from build123d import *

# Parameters (mm, degrees)
MODEL_R         = 0.5
MODEL_R_2       = 1.782992023
MODEL_R_3       = 1.590607237
MODEL_R_4       = 1.168321926
MODEL_R_5       = 1.005990221
MODEL_R_6       = 0.862372678
MODEL_R_7       = 1.386768465
MODEL_R_8       = 2.007691982
MODEL_R_9       = 2.246211192
EXTRUDE_1_DEPTH = 2


with BuildPart() as part:
    # Model → 凸台-拉伸1 (new body)
    with BuildSketch(Plane.XY):
        with BuildLine():
            Line((7.038065488, 6.287794997), (6.161323194, 8.085383089))
            Line((6.161323194, 8.085383089), (11.554087472, 10.71560997))
            Line((11.554087472, 10.71560997), (12.430829766, 8.918021877))
            Line((12.430829766, 8.918021877), (22.753800963, 13.952871341))
            Line((22.753800963, 13.952871341), (27.429909526, 30.259640434))
            ThreePointArc((27.429909526, 30.259640434), (29.651920806, 31.70137695), (31.356032886, 29.673584966))
            Line((31.356032886, 29.673584966), (31.073854544, 12.913284736))
            Line((31.073854544, 12.913284736), (84.46937713, 7.138642034))
            Line((84.46937713, 7.138642034), (76.356996628, 7.138642034))
            Line((76.356996628, 7.138642034), (76.356996628, 5.138642034))
            Line((76.356996628, 5.138642034), (84.613173024, 5.138642034))
            Line((84.613173024, 5.138642034), (84.613173024, 3.138642034))
            Line((84.613173024, 3.138642034), (39.080128632, 2.952174352))
            Line((39.080128632, 2.952174352), (6.368039675, 2.818983184))
            Line((6.368039675, 2.818983184), (6.36396809, 3.818974895))
            Line((6.36396809, 3.818974895), (1.939296742, 3.800959318))
            Line((1.939296742, 3.800959318), (7.038065488, 6.287794997))
        make_face()
        with Locations((29.356650707, 29.723293138)):
            Circle(MODEL_R, mode=Mode.SUBTRACT)
        with Locations((34.697579439, 7.654463755)):
            Circle(MODEL_R_2, mode=Mode.SUBTRACT)
        with Locations((40.228196013, 7.265180246)):
            Circle(MODEL_R_3, mode=Mode.SUBTRACT)
        with Locations((57.662403713, 6.323039134)):
            Circle(MODEL_R_4, mode=Mode.SUBTRACT)
        with Locations((61.677618383, 6.049673892)):
            Circle(MODEL_R_5, mode=Mode.SUBTRACT)
        with Locations((65.97541766, 5.870473213)):
            Circle(MODEL_R_6, mode=Mode.SUBTRACT)
        with Locations((45.214294389, 6.944127982)):
            Circle(MODEL_R_7, mode=Mode.SUBTRACT)
        with Locations((28.636152213, 7.943525557)):
            Circle(MODEL_R_8, mode=Mode.SUBTRACT)
        with Locations((22.680090468, 8.022724278)):
            Circle(MODEL_R_9, mode=Mode.SUBTRACT)
        with Locations((51.523752732, 6.556908357)):
            Circle(MODEL_R_7, mode=Mode.SUBTRACT)
    extrude(amount=EXTRUDE_1_DEPTH)


solid = part.part
Could you check a few things on this model? Use its own coordinates, in mm. A direction names the side the tool comes from. Coordinates: 2 decimals unless noted, no trailing zeros. Loops run counter-clockwise (first coordinate to the right, second up) from the corner with the lowest first, then second, coordinate; pieces in that order, holes last.
1. For faces 4 (the face through (12, 9.8, 1)), 5 (the face through (76.357, 6, 1)), 6 (the face through (6.61, 7.17, 0.99)), which set-ups out of +Z, -Z, +X, -X, +Y, -Y let a thin tool reach every point of the face, with its end or its side?
2. For P1, Ø4.5, axis at x = 28.64, y = 7.94, coming from the -Z side; P2, Ø1, axis at x = 80.5, z = 0.5, coming from the -Y side; P3, Ø1, axis at y = 6.5, z = 1, coming from the +X side, each with a flat end and sliding along its axis, tell me the tip position at first contact or that it passes through.
3. Imagine slicing it at B-B (z = 1.2). Give the number of separate pieces and of enclosed holes in the cut face, and give its area (3 significant figures).
4. Imagine slicing it at D-D (x = 19.5). Please give me the cut outline in (y, z).
5. Imagine slicing it at A-A (x = 61.5). Please give me the cut outline in (y, z), and give its area (3 significant figures).
6. I need wall thicknesses on L1, parallel to Y at x = 29, z = 1.05; L2, parallel to Y at x = 46, z = 1.1; L3, parallel to Y at x = 35, z = 1.05. Which ranges of each line are inside material? Lowest first, please.
7. Imagine slicing it at C-C (y = 20.5). Please give me the cut outline in (x, z).
8. We'd pull the mould along Y, two halves only. Please class faces 1 (the face through (25.06, 21.99, 0.99)), 2 (the face through (26.63, 8.03, 0.99)), 3 (the face through (84.613, 4, 1)): released by +Y, released by -Y, zero draft, split by the parting line, or undercut.
Computed values:
1. face 4: +Z, -Z, +Y
1. face 5: +Z, -Z, +X
1. face 6: +Z, -Z, -X
2. P1: stops at z = 0
2. P2: stops at y = 3.12
2. P3: stops at x = 76.36
3. separate pieces: 1
3. enclosed holes: 10
3. area: 618 mm2
4. outline: (2.87, 0) - (12.37, 0) - (12.37, 2) - (2.87, 2) - close
5. outline: (3.04, 0) - (5.06, 0) - (5.06, 2) - (3.04, 2) - close; (7.04, 0) - (9.62, 0) - (9.62, 2) - (7.04, 2) - close
5. area: 9.20 mm2
6. L1: y = 2.91 to 5.97, 9.92 to 29.37, 30.07 to 31.69
6. L2: y = 2.98 to 5.8, 8.09 to 11.3
6. L3: y = 2.94 to 5.9, 9.41 to 12.49
7. outline: (24.63, 0) - (31.2, 0) - (31.2, 2) - (24.63, 2) - close
8. face 1: released by +Y
8. face 2: undercut
8. face 3: zero draft
